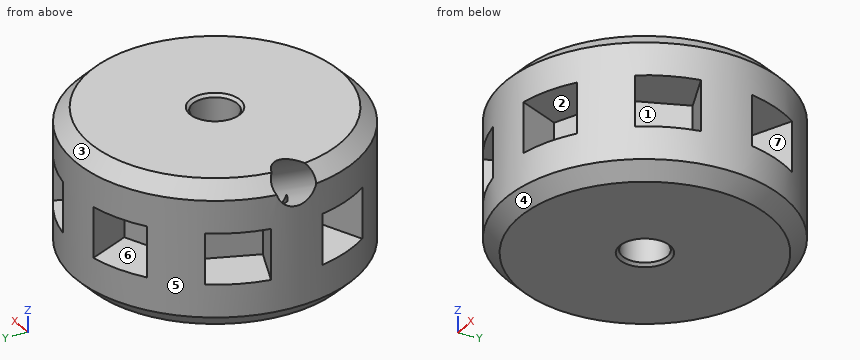
```python
from build123d import *

# Parameters (mm, degrees)
BOX001_W                = 4
BOX001_H                = 10
BOX001_DEPTH            = 3.5
BOX001_PLACEMENT_ANGLE  = 1
ARRAY_COUNT             = 8
ARRAY_PLACEMENT_ANGLE   = 22.5
CYLINDER004_R           = 1.45
CYLINDER004_DEPTH       = 50
CYLINDER004_PITCH_ANGLE = -60
CYLINDER002_R           = 1.55
CYLINDER002_DEPTH       = 20
CYLINDER_R              = 9.7
CYLINDER_DEPTH          = 10
CHAMFER_SIZE            = 1
CHAMFER001_SIZE         = 0.2


with BuildPart() as array:
    # Box001 → Box001 (new body)
    with BuildSketch(Plane.XY):
        with Locations((2, 5)):
            Rectangle(BOX001_W, BOX001_H)
    extrude(amount=BOX001_DEPTH)


with BuildPart() as array_1:
    # Box001 placement: moved
    add(array.part.moved(Location((-2, 6.3, 3.25))).rotate(Axis((-2, 6.3, 3.25), (0, 0, 1)), BOX001_PLACEMENT_ANGLE))

    # Array: Array ×8 about axis
    array_axis = Axis((0, 0, 0), (0, 0, 1))


with BuildPart() as array_2:
    add(array_1.part)
    for i in range(1, ARRAY_COUNT):
        add(array_1.part.rotate(array_axis, i * 360 / ARRAY_COUNT))


with BuildPart() as array_3:
    # Array placement: moved
    add(array_2.part.rotate(Axis((0, 0, 0), (0, 0, 1)), ARRAY_PLACEMENT_ANGLE))


with BuildPart() as tornillo:
    # Cylinder004 → Cylinder004 (new body)
    with BuildSketch(Plane.XY):
        Circle(CYLINDER004_R)
    extrude(amount=CYLINDER004_DEPTH)


with BuildPart() as tornillo_1:
    # Cylinder004 pitch: moved
    add(tornillo.part.rotate(Axis((0, 0, 0), (0, 1, 0)), CYLINDER004_PITCH_ANGLE))


with BuildPart() as tornillo_2:
    # Cylinder004 placement: moved
    add(tornillo_1.part.moved(Location((0, 0, 4))))


with BuildPart() as fusion:
    # Cylinder002 → Cylinder002 (new body)
    with BuildSketch(Plane.XY):
        Circle(CYLINDER002_R)
    extrude(amount=CYLINDER002_DEPTH)

    # Fusion: union Array, tornillo
    add(array_3.part)
    add(tornillo_2.part)


with BuildPart() as chamfer001:
    # Cylinder → Cylinder (new body)
    with BuildSketch(Plane.XY):
        Circle(CYLINDER_R)
    extrude(amount=CYLINDER_DEPTH)

    # Chamfer
    chamfer_edges = [chamfer001.edges().sort_by_distance(p)[0] for p in [
        (-9.7, 0, 10),
        (-9.7, 0, 0),
    ]]
    chamfer(chamfer_edges, length=CHAMFER_SIZE)

    # Cut: cut Fusion
    add(fusion.part, mode=Mode.SUBTRACT)

    # Chamfer001
    chamfer001_edges = [chamfer001.edges().sort_by_distance(p)[0] for p in [
        (-1.55, 0, 0),
        (-1.55, 0, 10),
    ]]
    chamfer(chamfer001_edges, length=CHAMFER001_SIZE)


solid = chamfer001.part
```
Could you check a few things on this model? Use its own coordinates, in mm. Face numbers are marked on the shaded views. A direction names the side the tool comes from. Give positions to 0.01 mm unless a question says otherwise; leave off trailing zeros. Order: outer loops, then holes, each group sorted by start corner. A loop starts at its lowest first (then second) coordinate and runs counter-clockwise, first axis right, second up.
Q1. I'm going to push flat-ended pins straight in: P1, Ø6, axis at x = -4.5, z = 7.5, coming from the +Y side; P2, Ø1.5, axis at x = 7, z = 5.5, coming from the -Y side; P3, Ø5, axis at x = 4.5, z = 8, coming from the -Y side. Where does each tip first touch, or does it pass through?
Q2. If I drill on line 1 along Y through (x, z) = (0, 4.5); line 2 along Z through (x, y) = (3, 5.75), over which ranges is the centre line in solid material (lowest first)?
Q3. For the marked faces 5, 6 and 7, which set-ups out of +Z, -Z, +X, -X, +Y, -Y let a thin tool reach every point of the face, with its end or its side?
Q4. We'd pull the mould along Z, two halves only. Please class the marked faces 1, 2, 3 and 4: +Z half, -Z half, draft (parallel to the pull), parting line (faces both ways), or undercut.
Q5. Suppose I cut it at B-B, the plane y = 0. Write out the boundary of the cut face in (x, z).
Q6. Suppose I cut it at A-A, the plane x = 0. Write out the boundary of the cut face in (y, z).
Solution:
1. P1: stops at y = 9.58
1. P2: stops at y = -7.42
1. P3: stops at y = -9.49
2. line 1: y = -9.7 to -1.55, 1.55 to 9.7
2. line 2: z = 0 to 3.25, 6.75 to 10
3. face 5: +Z, -Z
3. face 6: none
3. face 7: +X
4. face 1: undercut
4. face 2: undercut
4. face 3: +Z half
4. face 4: -Z half
5. outline: (-9.7, 1) - (-8.7, 0) - (-1.75, 0) - (-1.55, 0.2) - (-1.55, 3.22) - (-9.7, 7.93) - close; (-7.49, 10) - (-1.55, 6.57) - (-1.55, 9.8) - (-1.75, 10) - close; (1.55, 0.2) - (1.75, 0) - (8.7, 0) - (9.7, 1) - (9.7, 9) - (8.7, 10) - (1.75, 10) - (1.55, 9.8) - close
6. outline: (-9.7, 1) - (-8.7, 0) - (-1.75, 0) - (-1.55, 0.2) - (-1.55, 9.8) - (-1.75, 10) - (-8.7, 10) - (-9.7, 9) - close; (1.55, 0.2) - (1.75, 0) - (8.7, 0) - (9.7, 1) - (9.7, 9) - (8.7, 10) - (1.75, 10) - (1.55, 9.8) - close
